Autodesk Inventor part; units mm, degrees
ref_plane "YZ Plane" through (0, 0, 0) normal (1, 0, 0) x (0, 1, 0)
ref_plane "XZ Plane" through (0, 0, 0) normal (0, 1, 0) x (-1, 0, 0)
ref_plane "XY Plane" through (0, 0, 0) normal (0, 0, 1) x (1, 0, 0)
sketch "Sketch1" plane through (0, 0, 0) normal (0, 1, 0) x (-1, 0, 0)
  line L0 (-10, 95) -> (10, 95)
  line L1 (10, 95) -> (10, -95)
  line L2 (10, -95) -> (-10, -95)
  line L3 (-10, -95) -> (-10, 95)
  line L4 (-10, 95) -> (10, -95) construction
  line L5 (10, 95) -> (-10, -95) construction
  line L6 (20, -95) -> (-20, -95)
  line L7 (-20, -95) -> (-20, -75)
  line L8 (-20, -75) -> (20, -75)
  line L9 (20, -75) -> (20, -95)
  line L10 (-20, 95) -> (20, 95)
  line L11 (20, 95) -> (20, 75)
  line L12 (20, 75) -> (-20, 75)
  line L13 (-20, 75) -> (-20, 95)
  point P0 (0, 0)
  point P1 (-10, 75)
  point P2 (-10, -75)
  point P3 (10, -75)
  point P4 (10, 75)
  dimension "d0" = 20
  dimension "d1" = 190
  dimension "d2" = 40
  dimension "d3" = 20
  dimension "d4" = 40
  dimension "d5" = 20
extrude "Extrusion1" add sketch "Sketch1" along normal blind 10
sketch "Sketch2" plane through (0, 10, 0) normal (0, 1, 0) x (1, 0, 0)
  circle A0 centre (0, 0) radius 23.5
  circle A1 centre (0, 0) radius 33.5
  dimension "d8" = 47
  dimension "d9" = 67
extrude "Extrusion2" add sketch "Sketch2" against normal blind 10
sketch "Sketch3" plane through (0, 10, 0) normal (0, 1, 0) x (1, 0, 0)
  circle A0 centre (0, 0) radius 23.5
extrude "Extrusion3" cut sketch "Sketch3" against normal blind 10
sketch "Sketch4" plane through (0, 10, 0) normal (0, 1, 0) x (1, 0, 0)
  circle A0 centre (-15, -85) radius 2
  circle A1 centre (15, -85) radius 2
  circle A2 centre (-15, 85) radius 2
  circle A3 centre (15, 85) radius 2
  point P0 (0, 0)
  dimension "d14" = 4
  dimension "d15" = 4
  dimension "d16" = 4
  dimension "d17" = 4
extrude "Extrusion4" cut sketch "Sketch4" against normal blind 10
sketch "Sketch5" plane through (0, 10, 0) normal (0, 1, 0) x (1, 0, 0)
  line L0 (24.2968, 4) -> (32.2968, 4)
  line L1 (32.2968, 4) -> (32.2968, -4)
  line L2 (32.2968, -4) -> (24.2968, -4)
  line L3 (24.2968, -4) -> (24.2968, 4)
  line L4 (24.2968, 4) -> (32.2968, -4) construction
  line L5 (32.2968, 4) -> (24.2968, -4) construction
  line L6 (-32.2968, -4) -> (-32.2968, 4)
  line L7 (-32.2968, 4) -> (-24.2968, 4)
  line L8 (-24.2968, 4) -> (-24.2968, -4)
  line L9 (-24.2968, -4) -> (-32.2968, -4)
  point P0 (0, 0)
  point P1 (28.2968, 0)
  point P2 (-28.2968, 0)
  dimension "d20" = 8
  dimension "d21" = 8
  dimension "d24" = 360
extrude "Extrusion5" add sketch "Sketch5" along normal blind 6
sketch "Sketch6" plane through (0, 16, 0) normal (0, 1, 0) x (1, 0, 0)
  line L0 (24.2968, 4) -> (24.2968, -4)
  line L1 (32.2968, 4) -> (24.2968, 4)
  line L2 (24.2968, 4) -> (24.2968, -4)
  line L3 (24.2968, -4) -> (32.2968, -4)
  line L4 (32.2968, -4) -> (32.2968, 4)
  circle A0 centre (28.2968, 0) radius 1.5
  circle A1 centre (-28.2968, 0) radius 1.5
  point P0 (0, 0)
  dimension "d28" = 3
  dimension "d31" = 360
extrude "Extrusion6" cut sketch "Sketch6" against normal through all contours A0 | A1
properties part number "upper_grip"
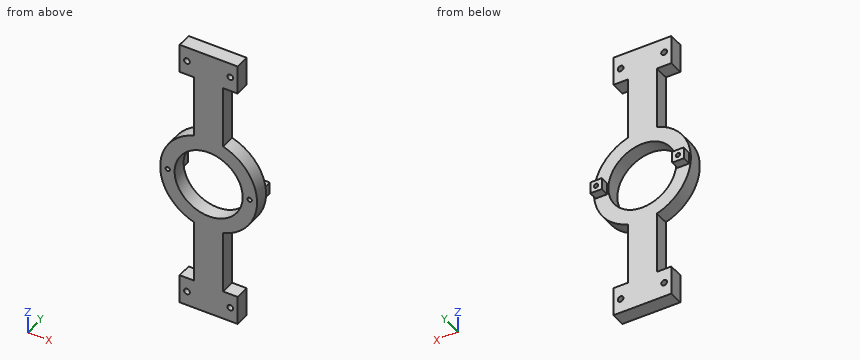
Input: part model. Units: mm. Frame: model coordinates. Give positions to 0.01 mm unless a question says otherwise; leave off trailing zeros. Write each loop counter-clockwise with the first axis right and the second up, starting at its lowest first coordinate (ties: lowest second). Pieces come first, ordered by that corner, then holes. Notation, with made-up numbers: (6.25, 86) -> (32.25, 86) arc R12 cw to (32.25, 107) -> close; hole circle Ø9 at (20, 9). An arc over 180 degrees is marked (long way). Use one line per item in the form item = value. Start each with the question number.
1) Section query A-A on y = 13.5. Return the cut outline in (x, z), then the cut area to 3 significant figures.
2) Section query C-C on x = 0. Return the cut outline in (y, z).
3) Section query D-D on y = 1.75. Return the cut outline in (x, z).
4) Ray query, probe 1 along X at (y, z) = (5.5, -85); probe 2 along Z at (x, y) = (15, 5.5); probe 3 along Z at (x, y) = (0, 7). Return the intervals inside material, ascending. Write a range as from..to.
5) Section query B-B on z = -85. Return the cut outline in (x, y).
6) Pin query (flat end, axial travel): pin 1 (6 mm diameter, centred on x = 2.5, y = 14, fed in from +Z); pin 2 (3 mm diameter, centred on y = 3.5, z = -43.5, fed in from +X); pin 3 (1.5 mm diameter, centred on x = -23, z = -8.5, fed in from +Y); pin 4 (8 mm diameter, centred on y = 6, z = -87, fed in from -X). Return the tip coordinate at first contact, or that it passes through.
Outcome:
q1.outline = (-32.3, -4) -> (-24.3, -4) -> (-24.3, 4) -> (-32.3, 4) -> close; (24.3, -4) -> (32.3, -4) -> (32.3, 4) -> (24.3, 4) -> close; hole circle Ø3 at (-28.3, 0); hole circle Ø3 at (28.3, 0)
q1.area = 114 mm^2
q2.outline = (0, -95) -> (10, -95) -> (10, -23.5) -> (0, -23.5) -> close; (0, 23.5) -> (10, 23.5) -> (10, 95) -> (0, 95) -> close
q3.outline = (-20, -95) -> (20, -95) -> (20, -75) -> (10, -75) -> (10, -31.97) arc R33.5 ccw to (10, 31.97) -> (10, 75) -> (20, 75) -> (20, 95) -> (-20, 95) -> (-20, 75) -> (-10, 75) -> (-10, 31.97) arc R33.5 ccw to (-10, -31.97) -> (-10, -75) -> (-20, -75) -> close; hole circle Ø3 at (-28.3, 0); hole circle Ø47 at (0, 0); hole circle Ø4 at (-15, -85); hole circle Ø4 at (-15, 85); hole circle Ø4 at (15, -85); hole circle Ø4 at (15, 85); hole circle Ø3 at (28.3, 0)
q4.probe_1 = -20..-17, -13..13, 17..20
q4.probe_2 = -95..-87, -83..-75, -29.95..-18.09, 18.09..29.95, 75..83, 87..95
q4.probe_3 = -95..-23.5, 23.5..95
q5.outline = (-20, 0) -> (-17, 0) -> (-17, 10) -> (-20, 10) -> close; (-13, 0) -> (13, 0) -> (13, 10) -> (-13, 10) -> close; (17, 0) -> (20, 0) -> (20, 10) -> (17, 10) -> close
q6.pin_1 = through
q6.pin_2 = 10
q6.pin_3 = 10
q6.pin_4 = -20
